Build history of the part. All positions in model axes, mm. A direction names the side the tool comes from. Give positions to 0.01 mm unless a question says otherwise; leave off trailing zeros. Loops run counter-clockwise (first coordinate to the right, second up) from the corner with the lowest first, then second, coordinate; pieces in that order, holes last.
1) Wall check: line 1 (X direction, y = 40, z = 11.75); line 2 (Y direction, x = 27.5, z = 2.25); line 3 (Y direction, x = 54, z = 4). Give the ranges that are in metal, low to high.
2) Two-plate mould, pull along Y, no slides. Class faces 3 (the cylindrical face through (-28.909, -241.345, 11.056)), 4 (the flat face through (-117.5, -3, 7)), 5 (the flat face through (-2, -250, 7)), 6 (the cylindrical face through (-58, 37, 7)): +Y half, -Y half, draft (parallel to the pull), parting line (faces both ways), or undercut.
3) 3-axis set-ups, long thin cutter, end or side, ignore diameter. For faces 1 (the flat face through (-27.6, -239.2, 7)), 2 (the flat face through (-2, 4, 0)): which of +Z, -Z, +X, -X, +Y, -Y reach the whole face in a straight line?
4) Band-saw the part on A-A on x = 54. List the corners of the cut face in (y, z).
5) Band-saw the part on B-B on y = 40. List the corners of the cut face in (x, z).
6) Flat gauge pin, fed straight in: P1, Ø4, axis at x = -30.5, y = -238, coming from the +Z side. Where does the tip first touch, or does it go through?
```python
from build123d import *

# Parameters (mm, degrees)
F0_W     = 235
F0_H     = 500
F1_DEPTH = 15
F2_R     = 4
F3_DEPTH = 25
F4_R     = 6.5
F5_DEPTH = 8
F6_R     = 5
F7_DEPTH = 15.001


with BuildPart() as f1:
    # F0 (on Top) → F1 (new body)
    with BuildSketch(Plane.XY):
        Rectangle(F0_W, F0_H)
    extrude(amount=F1_DEPTH)

    # F2 (on face) → F3 (cut)
    with BuildSketch(Plane.XY.offset(15)):
        with Locations((27.5, -235)):
            Circle(F2_R)
        with Locations((-27.5, -235)):
            Circle(F2_R)
    extrude(amount=-F3_DEPTH, mode=Mode.SUBTRACT)

    # F4 (on face) → F5 (cut)
    with BuildSketch(Plane.XY.offset(15)):
        with Locations((27.5, -235)):
            Circle(F4_R)
        with Locations((-27.5, -235)):
            Circle(F4_R)
    extrude(amount=-F5_DEPTH, mode=Mode.SUBTRACT)

    # F6 (on face) → F7 (cut, through all)
    with BuildSketch(Plane(origin=(0, 0, 0), x_dir=(1, 0, 0), z_dir=(0, 0, -1))):
        with Locations((54, -40)):
            Circle(F6_R)
        with Locations((-54, -40)):
            Circle(F6_R)
    extrude(amount=-F7_DEPTH, mode=Mode.SUBTRACT)


solid = f1.part
```
Findings below:
1. line 1: x = -117.5 to -59, -49 to 49, 59 to 117.5
1. line 2: y = -250 to -239, -231 to 250
1. line 3: y = -250 to 35, 45 to 250
2. face 3: undercut
2. face 4: draft
2. face 5: -Y half
2. face 6: undercut
3. face 1: +Z
3. face 2: -Z, +X, -X, +Y, -Y
4. outline: (-250, 0) - (35, 0) - (35, 15) - (-250, 15) - close; (45, 0) - (250, 0) - (250, 15) - (45, 15) - close
5. outline: (-117.5, 0) - (-59, 0) - (-59, 15) - (-117.5, 15) - close; (-49, 0) - (49, 0) - (49, 15) - (-49, 15) - close; (59, 0) - (117.5, 0) - (117.5, 15) - (59, 15) - close
6. P1: stops at z = 7
